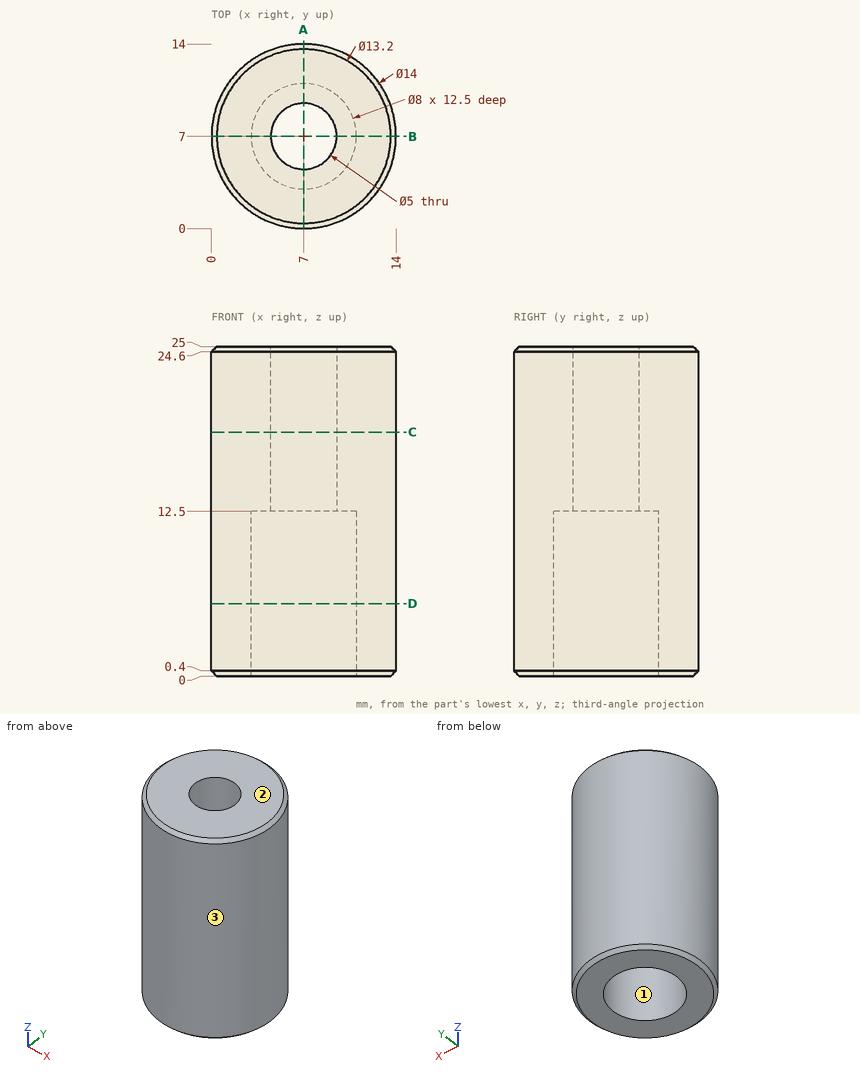
Study the drawing (mm; zero at the part's minimum x, y, z) and answer. Give positions to 0.01 mm unless a question says otherwise; leave off trailing zeros. Write each loop counter-clockwise with the first axis right and the second up, starting at its lowest first coordinate (ties: lowest second). Pieces come first, ordered by that corner, then holes. Notation, with made-up numbers: (50, -24) - (108, -24) arc R9 ccw to (108, -7) - close; hole circle Ø9 at (-1, 14). An arc over 180 degrees is marked (long way). One line per question, with ' | ' between items. Start each with the question number.
1. Determine the mould class of the marked faces 1, 2 and 3 for opening direction Y: +Y half, -Y half, draft (parallel to the pull), parting line (faces both ways), or undercut.
2. Given P1, Ø7, axis at x = 7, y = 7, coming from the -Z side; P2, Ø8, axis at y = 10, z = 15, coming from the -X side; P3, Ø2, axis at y = 9, z = 20, coming from the -X side, each flat-ended and moving along its own axis, determine where each tip first touches the part or whether it passes through.
3. Section D-D, the plane z = 5.5 is taken. Determine the outline of the cut face in (x, y), then the cut area to 3 significant figures.
4. Section C-C, the plane z = 18.5 is taken. Determine the outline of the cut face in (x, y), then the cut area to 3 significant figures.
5. Straight lines are drawn through the part: line 1 (Y direction, x = 7, z = 2.75); line 2 (Z direction, x = 9, y = 10); line 3 (X direction, y = 4.5, z = 8.5). For each, find the intervals that lie inside material, in ascending order.
6. Section A-A, the plane x = 7 is taken. Determine the outline of the cut face in (y, z).
Result:
1) face 1: undercut | face 2: draft | face 3: parting line
2) P1: stops at z = 12.5 | P2: stops at x = 0 | P3: stops at x = 0.07
3) outline: circle Ø14 at (7, 7); hole circle Ø8 at (7, 7) | area: 104 mm2
4) outline: circle Ø14 at (7, 7); hole circle Ø5 at (7, 7) | area: 134 mm2
5) line 1: y = 0 to 3, 11 to 14 | line 2: z = 12.5 to 25 | line 3: x = 0.46 to 3.88, 10.12 to 13.54
6) outline: (0, 0.4) - (0.4, 0) - (3, 0) - (3, 12.5) - (4.5, 12.5) - (4.5, 25) - (0.4, 25) - (0, 24.6) - close; (9.5, 12.5) - (11, 12.5) - (11, 0) - (13.6, 0) - (14, 0.4) - (14, 24.6) - (13.6, 25) - (9.5, 25) - close
